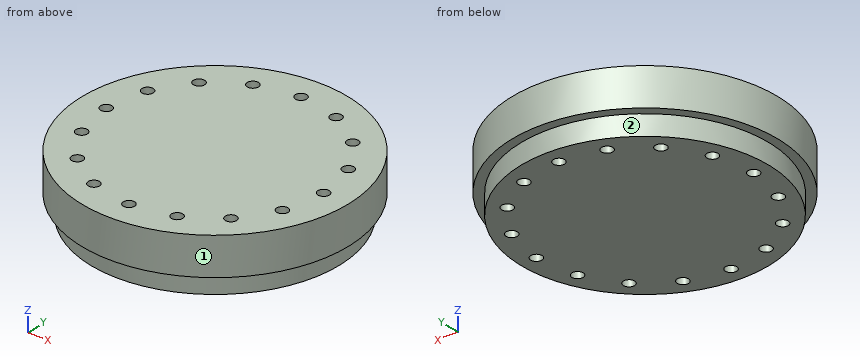
from build123d import *

# Parameters (mm, degrees)
SKETCH1_R           = 29.5
BOSS_EXTRUDE1_DEPTH = 4.175
SKETCH2_R           = 27.5
BOSS_EXTRUDE2_DEPTH = 4.45
SKETCH3_R           = 1.25
CUT_EXTRUDE1_DEPTH  = 44.638744253
CIRPATTERN1_COUNT   = 16


with BuildPart() as part:
    # Sketch1 → Boss-Extrude1 (new, symmetric)
    with BuildSketch(Plane.XY):
        Circle(SKETCH1_R)
    extrude(amount=BOSS_EXTRUDE1_DEPTH, both=True)

    # Sketch2 → Boss-Extrude2 (add)
    with BuildSketch(Plane(origin=(0, 0, -4.175), x_dir=(-1, 0, 0), z_dir=(0, 0, -1))):
        Circle(SKETCH2_R)
    extrude(amount=BOSS_EXTRUDE2_DEPTH)

    # Sketch3 → Cut-Extrude1 (cut, through all)
    with BuildSketch(Plane.XY.offset(4.175)):
        with Locations((0, 23.75)):
            Circle(SKETCH3_R)
    cut_extrude1 = extrude(amount=-CUT_EXTRUDE1_DEPTH, mode=Mode.SUBTRACT)

    # CirPattern1: Cut-Extrude1 ×16 about axis
    cirpattern1_axis = Axis((0, 0, 0), (0, 0, 1))
    for i in range(1, CIRPATTERN1_COUNT):
        add(cut_extrude1.rotate(cirpattern1_axis, i * 360 / CIRPATTERN1_COUNT), mode=Mode.SUBTRACT)


solid = part.part
Work out the finished part from the listing and answer in its coordinate system (mm). Face numbers are marked on the shaded views. A direction names the side the tool comes from. Round coordinates to 2 decimals unless told otherwise and drop trailing zeros. Loops run counter-clockwise (first coordinate to the right, second up) from the corner with the lowest first, then second, coordinate; pieces in that order, holes last. Notation, with made-up numbers: (1.5, -28) - (60.5, -28) arc R32 cw to (60.5, 5) - close; hole circle Ø5 at (65, 21). An arc over 180 degrees is marked (long way). One line per item, written item: value.
Q1. For the marked faces 1 and 2, determine the directions among +Z, -Z, +X, -X, +Y, -Y from which every point of the face is accessible in a straight line to the end or side of a thin tool.
Check values:
face 1: +Z, -Z
face 2: -Z
Q2. Find section D-D on y = -11.5. Give the vertices of the cut face in (x, z) (3 decimals).
Check values:
outline: (-27.166, -4.175) - (-24.98, -4.175) - (-24.98, -8.625) - (24.98, -8.625) - (24.98, -4.175) - (27.166, -4.175) - (27.166, 4.175) - (-27.166, 4.175) - close
Q3. Straight lines are drawn through the part: probe 1 along Y at (x, z) = (0, -4.5); probe 2 along Y at (x, z) = (0, -0.5); probe 3 along X at (y, z) = (-8.5, 2.25). For each, find the intervals that lie inside material, in ascending order.
Check values:
probe 1: -27.5 to -25, -22.5 to 22.5, 25 to 27.5
probe 2: -29.5 to -25, -22.5 to 22.5, 25 to 29.5
probe 3: -28.25 to -23.04, -20.84 to 20.84, 23.04 to 28.25
Q4. Each of these flat-tipped pins is pushed along its axis until it touches: pin 1 Ø3 at (x, z) = (0.5, -6) entering from -Y; pin 2 Ø1.5 at (x, y) = (16.79, -16.79) entering from -Z; pin 3 Ø5 at (x, z) = (-11, -2) entering from -Y; pin 4 Ø1 at (x, z) = (19, -0.5) entering from +Y. Where does it stop, or does it pass through?
Check values:
pin 1: y = -27.5
pin 2: through
pin 3: y = -28.25
pin 4: y = 22.98
Q5. Find section A-A on y = 0. Give the vertices of the cut face in (x, z) (3 decimals).
Check values:
outline: (-29.5, -4.175) - (-27.5, -4.175) - (-27.5, -8.625) - (-25, -8.625) - (-25, 4.175) - (-29.5, 4.175) - close; (-22.5, -8.625) - (22.5, -8.625) - (22.5, 4.175) - (-22.5, 4.175) - close; (25, -8.625) - (27.5, -8.625) - (27.5, -4.175) - (29.5, -4.175) - (29.5, 4.175) - (25, 4.175) - close
Q6. Find section C-C on z = 0.5. State how many separate pieces and enclosed holes the cut face has, and give its area (3 significant figures).
Check values:
separate pieces: 1
enclosed holes: 16
area: 2,660 mm2
